Part print with two shaded views. Sizes in mm from the minimum x, y, z corner. A direction names the side the tool comes from. Round coordinates to 2 decimals unless told otherwise and drop trailing zeros. Order: outer loops, then holes, each group sorted by start corner. A loop starts at its lowest first (then second) coordinate and runs counter-clockwise, first axis right, second up. Notation, with made-up numbers: (69, 79.5) -> (78, 79.5) arc R27 cw to (78, 106.5) -> close; hole circle Ø5 at (40, -18). An arc over 180 degrees is marked (long way). Use a Markdown table: item, result. Add a question column.
Item 1: Slice it at D-D, the plane x = 15. Give the cut face in (y, z).
Item 2: Probe L1, parallel to X at y = 2.5, z = 10; L2, parallel to X at y = 6, z = 10; L3, parallel to Y at x = 19.5, z = 14.5 (1 decimal). List the from-to ranges inside material, lowest first.
Item 3: Slice it at A-A, the plane z = 10. State how many separate pieces and enclosed holes the cut face has, plus the area to 3 significant figures.
Item 4: Slice it at B-B, the plane z = 18.25. Give the cut face in (x, y) (1 decimal).
Item 5: Slice it at C-C, the plane y = 27. Give the cut face in (x, z), plus the area to 3 significant figures.
Item 6: Pin check, flat tips, straight feed: pin 1 (10 mm diameter, centred on y = 16.5, z = 5, fed in from +X); pin 2 (1.5 mm diameter, centred on x = 15, z = 10, fed in from +Y); pin 3 (8 mm diameter, centred on x = 45, z = 6.5, fed in from +Y). Stop position of each tip, or through.
Item 7: 3-axis set-ups, long thin cutter, end or side, ignore diameter. For the marked faces 1 and 2: which of +Z, -Z, +X, -X, +Y, -Y reach the whole face in a straight line?
Item 8: Two-plate mould, pull along Z, no slides. Class the marked faces 3, 4 and 5: released by +Z, released by -Z, zero draft, split by the parting line, or undercut.
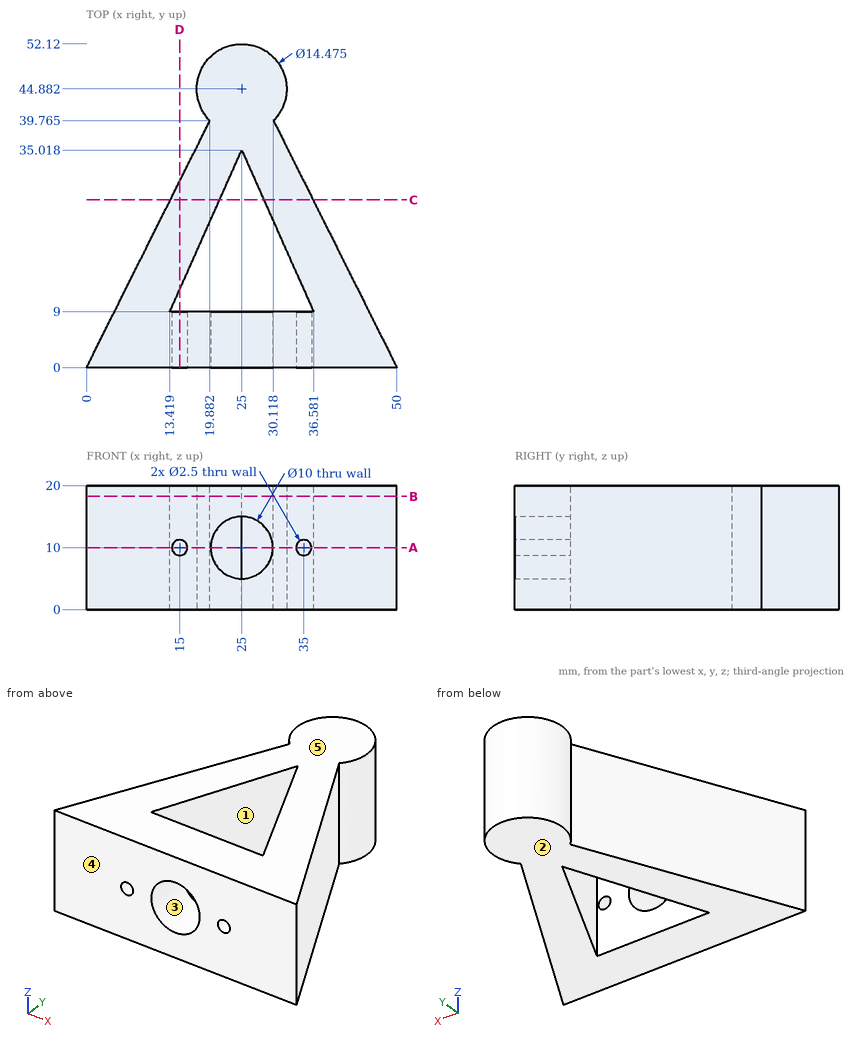
Check sheet entries:
| question | item | result |
|---|---|---|
| 1 | outline | (0, 0) -> (9, 0) -> (9, 8.75) -> (0, 8.75) -> close; (0, 11.25) -> (9, 11.25) -> (9, 20) -> (0, 20) -> close; (12.55, 0) -> (30, 0) -> (30, 20) -> (12.55, 20) -> close |
| 2 | L1 | 1.25 to 13.75, 16.25 to 20, 30 to 33.75, 36.25 to 48.75 |
| 2 | L2 | 3 to 13.75, 16.25 to 20, 30 to 33.75, 36.25 to 47 |
| 2 | L3 | 0 to 9, 22.7 to 39, 40.2 to 49.6 |
| 3 | separate pieces | 3 |
| 3 | enclosed holes | 0 |
| 3 | area | 911 mm2 |
| 4 | outline | (0, 0) -> (50, 0) -> (30.1, 39.8) arc R7.2 ccw (long way) to (19.9, 39.8) -> close; hole (13.4, 9) -> (36.6, 9) -> (25, 35) -> close |
| 5 | outline | (13.5, 0) -> (21.43, 0) -> (21.43, 20) -> (13.5, 20) -> close; (28.57, 0) -> (36.5, 0) -> (36.5, 20) -> (28.57, 20) -> close |
| 5 | area | 317 mm2 |
| 6 | pin 1 | x = 44.25 |
| 6 | pin 2 | y = 31.5 |
| 6 | pin 3 | y = 18 |
| 7 | face 1 | +Z, -Z |
| 7 | face 2 | -Z, +X, -X, +Y, -Y |
| 8 | face 3 | undercut |
| 8 | face 4 | zero draft |
| 8 | face 5 | released by +Z |
